Autodesk Inventor part; units mm, degrees
ref_plane "YZ Plane" through (0, 0, 0) normal (1, 0, 0) x (0, 1, 0)
ref_plane "XZ Plane" through (0, 0, 0) normal (0, 1, 0) x (-1, 0, 0)
ref_plane "XY Plane" through (0, 0, 0) normal (0, 0, 1) x (1, 0, 0)
sketch "スケッチ1" plane through (0, 0, 0) normal (1, 0, 0) x (0, 1, 0)
  line L0 (10, -90) -> (-10, -90)
  line L1 (-10, -90) -> (-10, 90)
  line L2 (-10, 90) -> (10, 90)
  line L3 (10, 90) -> (10, -90)
  line L4 (10, -90) -> (-10, 90) construction
  line L5 (-10, -90) -> (10, 90) construction
  point P0 (0, 0)
  dimension "d0" = 180
  dimension "d1" = 20
extrude "押し出し1" add sketch "スケッチ1" along normal blind 8
sketch "スケッチ2" plane through (8, 0, 0) normal (1, 0, 0) x (0, 0, -1)
  line L0 (-90, 10) -> (-90, -10)
  line L1 (90, -10) -> (90, 10)
  point P0 (0, 0)
  point P1 (-80, 0)
  point P2 (80, 0)
  dimension "d4" = 10
  dimension "d14" = 10
hole "穴1" at (8, 0, 80) at (8, 0, -80) direction (-1, 0, 0) diameter 12.3 end through all
fillet "フィレット1" radius 10 4 edges at (4, 10, 90) (4, -10, 90) (4, 10, -90) (4, -10, -90)
fillet "フィレット2" radius 1 8 edges at (0, 7.0712, -87.0712) (0, 10, 0) (0, 7.0712, 87.0712) (0, -10, 0) (8, 7.0712, -87.0712) (8, 10, 0) (8, 7.0712, 87.0712) (8, -10, 0)
properties part number "base4" material "ABS プラスチック"
CAD build for the part. Positions are in the model's coordinates, mm. Round coordinates to 2 decimals unless told otherwise and drop trailing zeros.
(1) Wall check: line 1 along Z through (x, y) = (6, 0); line 2 along Y through (x, z) = (2.25, 80); line 3 along Z through (x, y) = (5, -2). Give the ranges that are in metal, low to high.
(2) Two-plate mould, pull along Y, no slides. Class faces 1 (the cylindrical face through (4.04, -6.99, 87.15)), 2 (the cylindrical face through (3.944, -1.847, 74.134)), 3 (the flat face through (0, 0, 1)), 4 (the cylindrical face through (3.944, -1.847, -85.866)): +Y half, -Y half, draft (parallel to the pull), parting line (faces both ways), or undercut.
(3) Cut at A-A (x = 5). State how many separate pieces and enclosed holes the cut face has, plus the area to 3 significant figures.
Findings below:
1. line 1: z = -90 to -86.15, -73.85 to 73.85, 86.15 to 90
1. line 2: y = -10 to -6.15, 6.15 to 10
1. line 3: z = -89.8 to -85.82, -74.18 to 74.18, 85.82 to 89.8
2. face 1: -Y half
2. face 2: undercut
2. face 3: draft
2. face 4: undercut
3. separate pieces: 1
3. enclosed holes: 2
3. area: 3,280 mm2
